Geometry check sheet. Reference: the model listing, model coordinates, mm. A direction names the side the tool comes from. Coordinates: 2 decimals unless noted, no trailing zeros. Return JSON: item names as keys, results as strings. Group by question number.
Item 1: Draft check along Z on faces 1 (the cylindrical face through (-3.07, 5.01, -5.62)), 2 (the flat face through (-3, 15, 0)), 3 (the flat face through (-1.905, 35, -3)). Enter one of: pulls with the +Z half, pulls with the -Z half, needs draft (parallel to the pull), parting line crosses it, or undercut.
Item 2: Gauge pin test, flat ends, axial feed: pin 1 (2 mm diameter, centred on y = 20, z = -4.5, fed in from -X); pin 2 (1.7 mm diameter, centred on y = 33.5, z = -2, fed in from +X); pin 3 (3 mm diameter, centred on y = 12.5, z = -4, fed in from -X). Record the tip position at first contact, or that the pin passes through.
Item 3: Tool access check on faces 4 (the flat face through (-3.683, 35, -3)), 5 (the flat face through (-3, 0, -6)), 6 (the flat face through (-3, 10.16, -4)). Record the directions out of +Z, -Z, +X, -X, +Y, -Y that give a thin tool (end or side, any length) a straight path to the whole face; none if there is none.
Item 4: Scan lines: probe 1 along Y at (x, z) = (-2.6, -5); probe 2 along Y at (x, z) = (-3.3, -1); probe 3 along Z at (x, y) = (-3.15, 8.5). Record each from-to range of solid material in increasing order.
Autodesk Inventor part; units mm, degrees
ref_plane "Work Plane1" through (0, 38.1, 0) normal (0, 1, 0) x (-1, 0, 0)
ref_plane "YZ Plane" through (0, 0, 0) normal (1, 0, 0) x (0, 1, 0)
ref_plane "XY Plane" through (0, 0, 0) normal (0, 0, 1) x (1, 0, 0)
sketch "Sketch6" plane through (0, 0, 0) normal (0, 1, 0) x (-1, 0, 0)
  line L0 (0, 0) -> (5.588, 0)
  line L1 (5.588, 0) -> (5.588, -6.35)
  line L2 (5.588, -6.35) -> (0, -6.35)
  line L3 (0, -6.35) -> (0, 0)
  arc A0 (0, -6.35) -> (5.588, -6.35) centre (2.794, -6.35) ccw
  dimension "d25" = 5.588
  dimension "d26" = 6.35
ref_plane "Work Plane1" through (0, 38.1, 0) normal (0, 1, 0) x (-1, 0, 0)
sketch "Sketch8" plane through (0, 38.1, 0) normal (0, 1, 0) x (-1, 0, 0)
  line L0 (4.3815, 0) -> (1.2065, 0)
  line L1 (1.2065, 0) -> (1.2065, -3.81)
  line L2 (1.2065, -3.81) -> (4.3815, -3.81)
  line L3 (4.3815, -3.81) -> (4.3815, 0)
  arc A0 (1.2065, -3.81) -> (4.3815, -3.81) centre (2.794, -3.81) ccw
  point P0 (0, 0)
  dimension "d27" = 3.175
  dimension "d28" = 3.81
  dimension "d49" = 1.2065
loft "Loft1" add profiles "Sketch6", "Sketch8"
sketch "Sketch9" plane through (-5.588, 0, 0) normal (0, 0, 1) x (1, 0, 0)
  line L0 (0, 0) -> (5.588, 0)
  line L1 (5.588, 0) -> (4.3815, 38.1)
  line L2 (1.2065, 38.1) -> (4.3815, 38.1)
  line L3 (0, 0) -> (1.2065, 38.1)
  line L4 (4.3815, 38.1) -> (5.588, 0)
  line L5 (4.5826, 31.75) -> (1.0054, 31.75)
  line L6 (0, 0) -> (1.2065, 38.1)
  dimension "d34" = 6.35
extrude "Extrusion5" add sketch "Sketch9" along normal blind 38.608 contours L3 L2 L1 L5
sketch "Sketch12" plane through (-2.794, 0, -6.35) normal (0, -1, 0) x (1, 0, 0)
  circle A0 centre (0, 1.9685) radius 1.27
  arc A1 (-2.794, 0) -> (2.794, 0) centre (0, 0) ccw
  line L0 (0, -2.794) -> (0, 1.9685)
  point P0 (2.794, 6.35)
  dimension "d44" = 2.54
  dimension "d46" = 4.7625
extrude "Extrusion8" cut sketch "Sketch12" against normal blind 10.16
sketch "Sketch13" plane through (-5.588, 0, 0) normal (0, 0, 1) x (1, 0, 0)
  line L0 (1.2065, 38.1) -> (4.3815, 38.1)
  line L1 (3.683, 38.1) -> (1.905, 38.1)
  line L2 (1.905, 38.1) -> (1.905, 31.75)
  line L3 (1.905, 31.75) -> (3.683, 31.75)
  line L4 (3.683, 31.75) -> (3.683, 38.1)
  line L5 (3.683, 31.75) -> (4.5826, 31.75) construction
  line L6 (4.3815, 38.1) -> (5.588, 0) construction
  line L7 (1.905, 31.75) -> (1.0054, 31.75) construction
  line L8 (0, 0) -> (1.2065, 38.1) construction
  line L9 (6.375, 40.676) -> (-2.8276, 40.676)
  line L10 (-2.8276, 40.676) -> (-2.8276, 26.7394)
  line L11 (-2.8276, 26.7394) -> (6.375, 26.7394)
  line L12 (6.375, 26.7394) -> (6.375, 40.676)
  dimension "d50" = 1.778
  dimension "d51" = 6.35
extrude "Extrusion9" cut sketch "Sketch13" against normal through all contours L0 L4 L3 L2
extrude "Extrusion10" cut sketch "Sketch13" along normal through all contours L0 L4 L3 L2 | L12 L11 L10 L9
properties part number "RudderStabilizingFinBottom_Print1"
Computed:
{
 "1": {"face 1": "undercut", "face 2": "pulls with the +Z half", "face 3": "needs draft"},
 "2": {"pin 1": "stops at x = -4.99", "pin 2": "stops at x = -1.03", "pin 3": "stops at x = -5.24"},
 "3": {"face 4": "+Z, -Z, +Y", "face 5": "+Z, -Z, +X, -X, -Y", "face 6": "-Y"},
 "4": {"probe 1": "y = 10.16 to 31.75", "probe 2": "y = 0 to 31.75", "probe 3": "z = -8.28 to -5.6, -3.16 to 0"}
}
